For this review, take the finished solid that the model builds, in its own axes (mm). A direction names the side the tool comes from. Coordinates: 2 decimals unless noted, no trailing zeros. Loops run counter-clockwise (first coordinate to the right, second up) from the corner with the lowest first, then second, coordinate; pieces in that order, holes last. Notation, with made-up numbers: M 22.25,5 L 43.25,5 A24 cw 43.25,25 Z; hole C 58,-34.75 d8. An arc over 180 degrees is marked long. Answer as a JSON object with one key per item and string values. Group by question number.
Item 1: Mouldability with a two-part tool opening along Y and no side actions: class faces 4 (the face through (28, 46, 12)), 5 (the face through (-0.661, 15.986, 27.608)), 6 (the face through (10.955, -25.768, 33.83)) as +Y half, -Y half, draft (parallel to the pull), parting line (faces both ways), or undercut.
Item 2: Insertion check: pin 1 (2 mm diameter, centred on y = -8, z = 23, fed in from +X); pin 2 (9.5 mm diameter, centred on y = -23, z = 15.5, fed in from -X); pin 3 (1.5 mm diameter, centred on x = 2.5, y = 49, fed in from +Z); pin 4 (17.5 mm diameter, centred on x = 5, z = 14, fed in from +Y). Each pin has a flat end and moves straight along its axis. Give the tip position at first contact, or say it passes through.
Item 3: Add section D-D (z = 17). State the section outline as (x, y) points.
Item 4: Tool access review of faces 1 (the face through (-3, -22, 28)), 2 (the face through (0, 70, 8)), 3 (the face through (12, -12, 56)): name each direction out of +Z, -Z, +X, -X, +Y, -Y from which nothing blocks a thin tool from reaching the whole face with its end or side.
Item 5: Add section B-B (y = -17.5). State the section outline as (x, z) points.
Item 6: Add section A-A (x = 6.5). State the section outline as (y, z) points.
Item 7: Add section C-C (x = 0). State the section outline as (y, z) points.
Item 8: Wall thickness on L1, parallel to X at y = 0, z = 26; L2, parallel to Z at x = -23, y = 77.5; L3, parallel to Y at x = -5, z = 25.5: over which ranges is each line inside the solid? List them lowest first. Write a range as from..to.
from build123d import *

# Parameters (mm, degrees)
BOSS_EXTRUDE1_DEPTH      = 56
BOSS_EXTRUDE2_REACH      = 135.439
BOSS_EXTRUDE2_END_RADIUS = 28
SKETCH2_W                = 56
SKETCH2_H                = 24
CUT_EXTRUDE1_DEPTH       = 40


with BuildPart() as part:
    # Sketch1 → Boss-Extrude1 (new body)
    with BuildSketch(Plane.XY):
        with BuildLine():
            Line((-3, -27.838821814), (-3, -15.716233646))
            ThreePointArc((-3, -15.716233646), (0, 16), (3, -15.716233646))
            Line((3, -15.716233646), (3, -27.838821814))
            ThreePointArc((3, -27.838821814), (0, 28), (-3, -27.838821814))
        make_face()
    extrude(amount=BOSS_EXTRUDE1_DEPTH)

    # Boss-Extrude2: up to this cylinder (the profile starts outside it)
    boss_extrude2_end = Plane(origin=(0, 0, 12), z_dir=(0, 0, -1)) * Cylinder(BOSS_EXTRUDE2_END_RADIUS, 327.878, mode=Mode.PRIVATE)
    # Sketch2 → Boss-Extrude2 (add, up to the surface)
    with BuildSketch(Plane(origin=(0, 90, 0), x_dir=(1, 0, 0), z_dir=(0, 1, 0)), mode=Mode.PRIVATE) as boss_extrude2_sk1:
        with Locations((0, -12)):
            Rectangle(SKETCH2_W, SKETCH2_H)
    boss_extrude2_tool1 = extrude(boss_extrude2_sk1.sketch, amount=-BOSS_EXTRUDE2_REACH, mode=Mode.PRIVATE) - boss_extrude2_end
    add(boss_extrude2_tool1.solids().sort_by_distance((0, 90, 12))[0])

    # Sketch3 → Cut-Extrude1 (cut)
    with BuildSketch(Plane(origin=(0, 90, 0), x_dir=(1, 0, 0), z_dir=(0, 1, 0))):
        with BuildLine():
            ThreePointArc((16, -24), (0, -8), (-16, -24))
            Line((-16, -24), (16, -24))
        make_face()
        with BuildLine():
            Line((16, -24), (-16, -24))
            ThreePointArc((-16, -24), (0, -40), (16, -24))
        make_face()
    extrude(amount=-CUT_EXTRUDE1_DEPTH, mode=Mode.SUBTRACT)


solid = part.part
From the geometry:
{
 "1": {"face 4": "draft", "face 5": "undercut", "face 6": "parting line"},
 "2": {"pin 1": "stops at x = 27.11", "pin 2": "stops at x = -21.24", "pin 3": "stops at z = 24", "pin 4": "stops at y = 90"},
 "3": {"outline": "M -28,0 A28 ccw -3,-27.84 L -3,-15.72 A16 cw long 3,-15.72 L 3,-27.84 A28 ccw 28,0 L 28,90 L 14.39,90 L 14.39,50 L -14.39,50 L -14.39,90 L -28,90 Z"},
 "4": {"face 1": "+Z, -Z, -Y", "face 2": "+Z, +Y", "face 3": "+Z, +X, -X, +Y, -Y"},
 "5": {"outline": "M -21.86,0 L -3,0 L -3,56 L -21.86,56 Z; M 3,0 L 21.86,0 L 21.86,56 L 3,56 Z"},
 "6": {"outline": "M -27.24,0 L -14.62,0 L -14.62,56 L -27.24,56 Z; M 14.62,0 L 90,0 L 90,9.38 L 50,9.38 L 50,24 L 27.24,24 L 27.24,56 L 14.62,56 Z"},
 "7": {"outline": "M 16,0 L 90,0 L 90,8 L 50,8 L 50,24 L 28,24 L 28,56 L 16,56 Z"},
 "8": {"L1": "x = -28..-16, 16..28", "L2": "z = 0..24", "L3": "y = -27.55..-15.2, 15.2..27.55"}
}
